from build123d import *

# Parameters (mm, degrees)
F2_SIZE2      = 10
F2_SIZE       = 10
F3_R          = 6
F4_DEPTH      = 40.001
F4_DEPTH_BACK = 40.001


with BuildPart() as f1:
    # F0 (on Top) → F1 (revolve)
    with BuildSketch(Plane.XY):
        Polygon((0, 40), (0, 0), (120, 0), (120, 18.0392161204), (30, 18.0392161204), (30, 40), align=None)
    revolve(axis=Axis((60, 0, 0), (-1, 0, 0)))

    # F2
    f2_edges = [f1.edges().sort_by_distance(p)[0] for p in [
        (0, -40, 0),
        (120, -18.039216, 0),
    ]]
    chamfer(f2_edges, length=F2_SIZE, length2=F2_SIZE2)

    # F3 (on Top) → F4 (cut, two sides)
    with BuildSketch(Plane.XY) as f4_sk:
        with Locations((102, 0)):
            Circle(F3_R)
    extrude(amount=-F4_DEPTH, mode=Mode.SUBTRACT)
    extrude(f4_sk.sketch, amount=F4_DEPTH_BACK, mode=Mode.SUBTRACT)


solid = f1.part
The listing builds one solid part. Answer for the finished solid, in the listing's coordinates (mm). A direction names the side the tool comes from. Give positions to 0.01 mm unless a question says otherwise; leave off trailing zeros. Write each loop counter-clockwise with the first axis right and the second up, starting at its lowest first coordinate (ties: lowest second). Pieces come first, ordered by that corner, then holes. Notation, with made-up numbers: (27, 31.25) - (60, 31.25) arc R22 cw to (60, 37.25) - close; hole circle Ø1 at (15, 27). An arc over 180 degrees is marked (long way). One line per question, with ' | ' between items. Start each with the question number.
1. For faces 1 (the face through (30, -17, 8)), 2 (the face through (120, 0, 0)), determine the directions among +Z, -Z, +X, -X, +Y, -Y from which every point of the face is accessible in a straight line to the end or side of a thin tool.
2. Straight lines are drawn through the part: line 1 (X direction, y = 0, z = -1); line 2 (Z direction, x = 18, y = 1); line 3 (X direction, y = -18.5, z = -23). For each, find the intervals that lie inside material, in ascending order.
3. Determine the mould class of faces 3 (the face through (0.626, -22.572, -20.698)), 4 (the face through (0, 0, 0)), 5 (the face through (96, 0, 0)) for opening direction Y: +Y half, -Y half, draft (parallel to the pull), parting line (faces both ways), or undercut.
4. Section B-B, the plane z = 0 is taken. Determine the outline of the cut face in (x, y).
5. Section A-A, the plane y = 0 is taken. Determine the outline of the cut face in (x, z).
6. Section C-C, the plane x = 69.5 is taken. Determine the outline of the cut face in (y, z), then the cut area to 3 significant figures.
7. Given P1, Ø6, axis at x = 103.5, y = 23, coming from the -Z side; P2, Ø4, axis at x = 93.5, y = 18, coming from the -Z side; P3, Ø8, axis at x = 49.5, z = -7.5, coming from the +Y side; P4, Ø4, axis at y = -5, z = -8, coming from the -X side, each flat-ended and moving along its own axis, determine where each tip first touches the part or whether it passes through.
8. Section D-D, the plane x = 102 is taken. Determine the outline of the cut face in (y, z).
Result:
1) face 1: +X | face 2: +Z, -Z, +X, +Y, -Y
2) line 1: x = 0 to 96, 108 to 120 | line 2: z = -39.99 to 39.99 | line 3: x = 0 to 30
3) face 3: parting line | face 4: draft | face 5: undercut
4) outline: (0, -30) - (10, -40) - (30, -40) - (30, -18.04) - (110, -18.04) - (120, -8.04) - (120, 8.04) - (110, 18.04) - (30, 18.04) - (30, 40) - (10, 40) - (0, 30) - close; hole circle Ø12 at (102, 0)
5) outline: (0, -30) - (10, -40) - (30, -40) - (30, -18.04) - (96, -18.04) - (96, 18.04) - (30, 18.04) - (30, 40) - (10, 40) - (0, 30) - close; (108, -18.04) - (110, -18.04) - (120, -8.04) - (120, 8.04) - (110, 18.04) - (108, 18.04) - close
6) outline: circle Ø36.08 at (0, 0) | area: 1,020 mm2
7) P1: passes through | P2: stops at z = -8.33 | P3: stops at y = 17.7 | P4: stops at x = 0
8) outline: (-6, -17.01) - (-6, 17.01) arc R18.04 ccw to start; (6, -17.01) arc R18.04 ccw to (6, 17.01) - close
